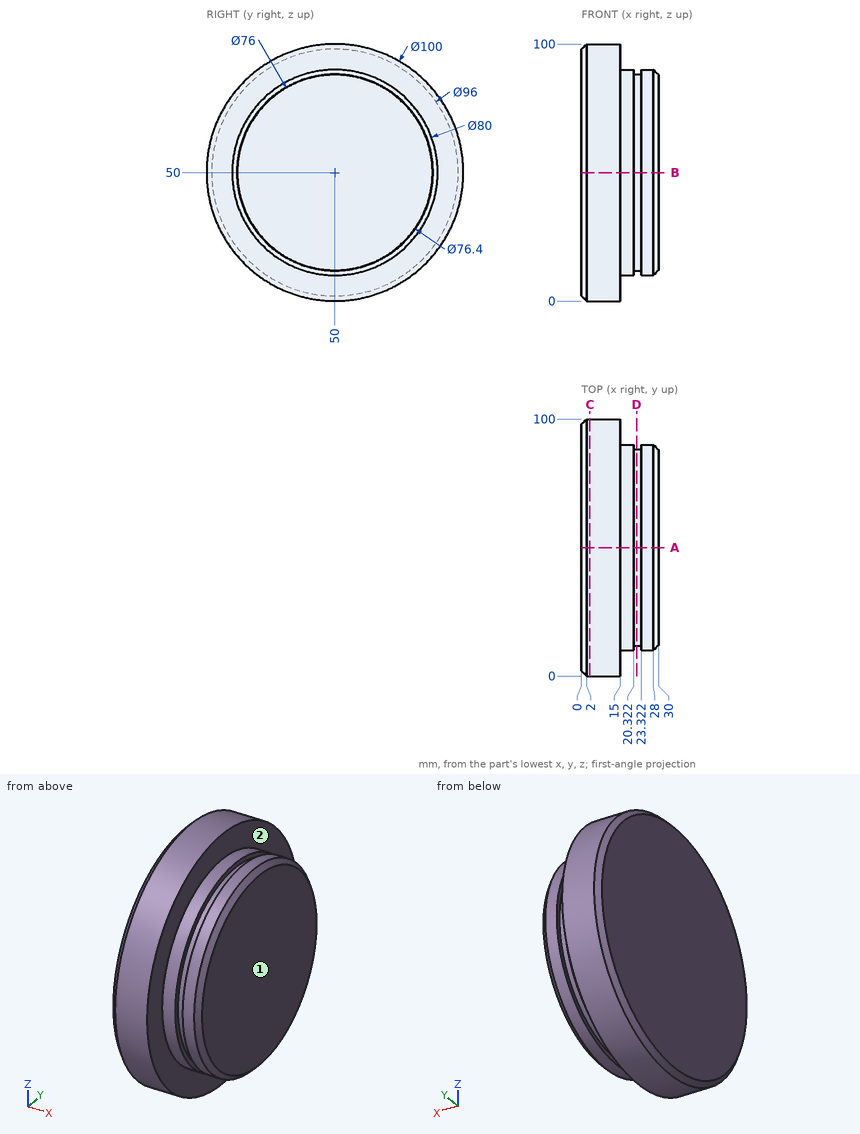
Input: dimensioned drawing with shaded views. Units: mm. Origin: part minimum x, y, z. A direction names the side the tool comes from. Give positions to 0.01 mm unless a question says otherwise; leave off trailing zeros. Write each loop counter-clockwise with the first axis right and the second up, starting at its lowest first coordinate (ties: lowest second). Pieces come first, ordered by that corner, then holes.
Q1. Section D-D, the plane x = 21.5. Output: boundary loops of the cut face in (y, z).
Q2. Section A-A, the plane y = 50. Output: boundary loops of the cut face in (x, z), plus the area to 3 significant figures.
Q3. Set-up query: the marked faces 1 and 2. Return all of +Z, -Z, +X, -X, +Y, -Y with unobstructed straight access to the full face (end or side cutting, diameter ignored); none if empty.
Q4. Section C-C, the plane x = 3.25. Output: boundary loops of the cut face in (y, z).
Q5. First-contact query: P1, Ø1, axis at x = 21.5, z = 53.5, coming from the -Y side; P2, Ø10, axis at x = 15, y = 24, coming from the +Z side; P3, Ø3, axis at x = 6, z = 17.5, coming from the +Y side. Flat tips, straight axial feed; report the tip coordinate or a pass-through.
Q6. Material intervals for probe 1 along X at (y, z) = (62.5, 94); probe 2 along Y at (x, z) = (7.5, 64); probe 3 along Y at (x, z) = (25.25, 74), sorted ascending.
Filled in:
1. outline: circle Ø76.4 at (50, 50)
2. outline: (0, 2) - (2, 0) - (15, 0) - (15, 10) - (20.32, 10) - (20.32, 11.8) - (23.32, 11.8) - (23.32, 10) - (28, 10) - (30, 12) - (30, 88) - (28, 90) - (23.32, 90) - (23.32, 88.2) - (20.32, 88.2) - (20.32, 90) - (15, 90) - (15, 100) - (2, 100) - (0, 98) - close
2. area: 2,680 mm2
3. face 1: +Z, -Z, +X, +Y, -Y
3. face 2: +X
4. outline: circle Ø100 at (50, 50)
5. P1: stops at y = 11.92
5. P2: stops at z = 95.38
5. P3: stops at y = 89.23
6. probe 1: x = 0 to 15
6. probe 2: y = 2 to 98
6. probe 3: y = 18 to 82
